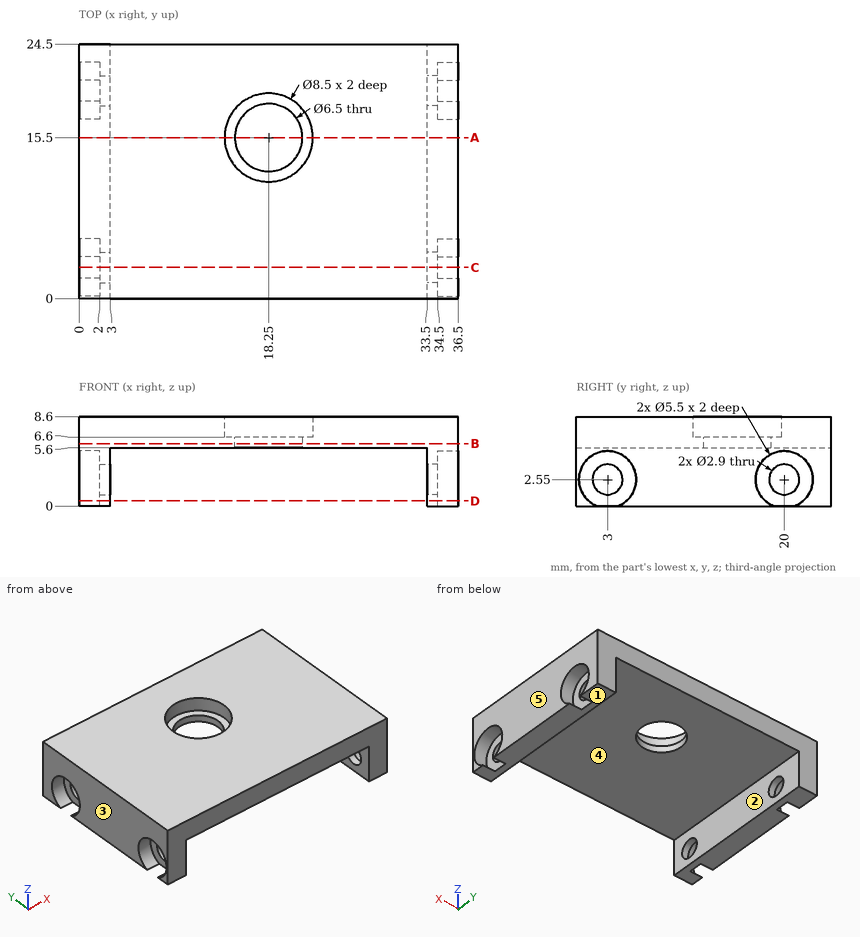
Design review of the part shown in the three views and the two pictorial views. Dimensions are in mm from the part's minimum x, y and z. A direction names the side the tool comes from. Give positions to 0.01 mm unless a question says otherwise; leave off trailing zeros. Write each loop counter-clockwise with the first axis right and the second up, starting at its lowest first coordinate (ties: lowest second). Pieces come first, ordered by that corner, then holes. Notation, with made-up numbers: M -12.5,16.25 L 17.5,16.25 A16 cw 17.5,37.25 Z; hole C 89.25,0.25 d10. An arc over 180 degrees is marked long. Answer as CSV lines item,"result".
1. For the marked faces 1 and 2, list the 3-axis set-ups (+Z, -Z, +X, -X, +Y, -Y) from which the entire face can be reached by the end or side of a thin tool; tool diameter is ignored.
Findings:
face 1,"-Z, +X, -X, +Y, -Y"
face 2,"-Z, +Y, -Y"
2. For pin 1 (5 mm diameter, centred on y = 20, z = 2.55, fed in from -X); pin 2 (2.5 mm diameter, centred on y = 3, z = 2.55, fed in from +X); pin 3 (12 mm diameter, centred on x = 17.5, y = 4, fed in from -Z), all flat-tipped, find the tip position at first contact; note any pin that passes through.
Findings:
pin 1,"stops at x = 2"
pin 2,"passes through"
pin 3,"stops at z = 5.6"
3. Consider section A-A, the plane y = 15.5. Write out the cut boundary in (x, z).
Findings:
outline,"M 0,0 L 3,0 L 3,5.6 L 15,5.6 L 15,6.6 L 14,6.6 L 14,8.6 L 0,8.6 Z; M 21.5,5.6 L 33.5,5.6 L 33.5,0 L 36.5,0 L 36.5,8.6 L 22.5,8.6 L 22.5,6.6 L 21.5,6.6 Z"
4. Consider section B-B, the plane z = 6. Write out the cut boundary in (x, y).
Findings:
outline,"M 0,0 L 36.5,0 L 36.5,24.5 L 0,24.5 Z; hole C 18.25,15.5 d6.5"
5. Wall thickness on line 1 (Y direction, x = 2.6, z = 2.55); line 2 (X direction, y = 20.75, z = 5.5); line 3 (X direction, y = 18, z = 3.5): over which ranges is each line inside the solid? List them lowest first.
Findings:
line 1,"y = 0 to 1.55, 4.45 to 18.55, 21.45 to 24.5"
line 2,"x = 0 to 3, 33.5 to 36.5"
line 3,"x = 2 to 3, 33.5 to 34.5"
6. Consider section D-D, the plane z = 0.5. Write out the cut boundary in (x, y).
Findings:
outline,"M 0,0 L 3,0 L 3,24.5 L 0,24.5 L 0,21.83 L 2,21.83 L 2,18.17 L 0,18.17 L 0,4.83 L 2,4.83 L 2,1.17 L 0,1.17 Z; M 33.5,0 L 36.5,0 L 36.5,1.17 L 34.5,1.17 L 34.5,4.83 L 36.5,4.83 L 36.5,18.17 L 34.5,18.17 L 34.5,21.83 L 36.5,21.83 L 36.5,24.5 L 33.5,24.5 Z"
7. Draft analysis for pull direction X (two halves, no side actions). For the marked faces 3, 4 and 5, state which applies: +X half, -X half, draft (parallel to the pull), parting line (faces both ways), or undercut.
Findings:
face 3,"-X half"
face 4,"undercut"
face 5,"+X half"
8. Consider section C-C, the plane y = 3. Write out the cut boundary in (x, z), then the cut area to 3 significant figures.
Findings:
outline,"M 0,5.3 L 2,5.3 L 2,4 L 3,4 L 3,5.6 L 33.5,5.6 L 33.5,4 L 34.5,4 L 34.5,5.3 L 36.5,5.3 L 36.5,8.6 L 0,8.6 Z; M 2,0 L 3,0 L 3,1.1 L 2,1.1 Z; M 33.5,0 L 34.5,0 L 34.5,1.1 L 33.5,1.1 Z"
area,"116 mm2"
